from build123d import *

# Parameters (mm, degrees)
BOSS_EXTRUDE1_DEPTH = 3.175
SKETCH2_R           = 2.032
CUT_EXTRUDE1_DEPTH  = 519.070111689


with BuildPart() as part:
    # Sketch1 → Boss-Extrude1 (new body)
    with BuildSketch(Plane(origin=(0, 0, 0), x_dir=(1, 0, 0), z_dir=(0, 1, 0))):
        with BuildLine():
            Line((0, 0), (0, -508))
            Line((0, -508), (101.6, -508))
            Line((101.6, -508), (101.6, 0))
            ThreePointArc((101.6, 0), (50.8, 25.4), (0, 0))
        make_face()
    extrude(amount=BOSS_EXTRUDE1_DEPTH)

    # Sketch2 → Cut-Extrude1 (cut, through all)
    with BuildSketch(Plane.XZ):
        with Locations(Location((21.59, 501.65, 0), (0, 0, 270))):
            Circle(SKETCH2_R)
        with Locations(Location((80.01, 501.65, 0), (0, 0, 270))):
            Circle(SKETCH2_R)
        with Locations(Location((21.59, 82.55, 0), (0, 0, 270))):
            Circle(SKETCH2_R)
        with Locations(Location((80.01, 82.55, 0), (0, 0, 270))):
            Circle(SKETCH2_R)
    extrude(amount=-CUT_EXTRUDE1_DEPTH, mode=Mode.SUBTRACT)


solid = part.part
CAD build for the part. Positions are in the model's coordinates, mm. Round coordinates to 2 decimals unless told otherwise and drop trailing zeros. Write each loop counter-clockwise with the first axis right and the second up, starting at its lowest first coordinate (ties: lowest second). Pieces come first, ordered by that corner, then holes.
(1) Slice it at C-C, the plane x = 91. Write the cut outline in (y, z) (3 decimals), and give its area (3 significant figures).
(2) Probe line 1 along X through (y, z) = (0.85, 82.55); line 2 along Z through (x, y) = (66.5, 0.9); line 3 along Z through (x, y) = (95.5, 1.8). List the from-to ranges inside material, lowest first.
(3) Slice it at B-B, the plane x = 14. Write the cut outline in (y, z) (1 decimal), and give its area (3 significant figures).
(4) Slice it at A-A, the plane y = 2.25. Write the cut outline in (x, z).
From the geometry:
1. outline: (0, -11.055) - (3.175, -11.055) - (3.175, 508) - (0, 508) - close
1. area: 1,650 mm2
2. line 1: x = 0 to 19.56, 23.62 to 77.98, 82.04 to 101.6
2. line 2: z = -23.43 to 508
2. line 3: z = -7 to 508
3. outline: (0, -13.6) - (3.2, -13.6) - (3.2, 508) - (0, 508) - close
3. area: 1,660 mm2
4. outline: (0, 0) arc R63.5 ccw to (101.6, 0) - (101.6, 508) - (0, 508) - close; hole circle Ø4.06 at (21.59, 82.55); hole circle Ø4.06 at (21.59, 501.65); hole circle Ø4.06 at (80.01, 82.55); hole circle Ø4.06 at (80.01, 501.65)
